Geometry: final body of the model. Coordinates: model frame, mm. A direction names the side the tool comes from. Give positions to 0.01 mm unless a question says otherwise; leave off trailing zeros. Order: outer loops, then holes, each group sorted by start corner. A loop starts at its lowest first (then second) coordinate and runs counter-clockwise, first axis right, second up. Notation, with made-up numbers: (58, 44.25) -> (65, 44.25) arc R14 cw to (65, 53.25) -> close; hole circle Ø4 at (76, 13.25). An arc over 180 degrees is marked (long way). One line per question, with ' | ' between items.
from build123d import *

# Parameters (mm, degrees)
BOSS_EXTRUDE1_DEPTH   = 3.175
BOSS_EXTRUDE1_2_DEPTH = 3.175
BOSS_EXTRUDE1_3_DEPTH = 3.175
BOSS_EXTRUDE1_4_DEPTH = 3.175
SKETCH1_R             = 3.2
SKETCH1_W             = 12.5
SKETCH1_H             = 20
BOSS_EXTRUDE1_5_DEPTH = 3.175
SKETCH2_W             = 43.267164734
SKETCH2_H             = 48
SKETCH2_W_2           = 36.488078293
BOSS_EXTRUDE2_DEPTH   = 3.175
SKETCH3_W             = 150
SKETCH3_H             = 50.164895034
SKETCH3_W_2           = 146
SKETCH3_H_2           = 48
BOSS_EXTRUDE3_DEPTH   = 3.175
SKETCH4_R             = 3.175
CUT_EXTRUDE1_DEPTH    = 3.175


with BuildPart() as part:
    # Sketch1 → Boss-Extrude1 (new body)
    with BuildSketch(Plane.XY):
        Polygon((57.693747285, -13.75), (57.693747285, -24), (73, -24), (73, -10.75), (53.098076211, -10.75), (53.098076211, -13.75), align=None)
    extrude(amount=BOSS_EXTRUDE1_DEPTH)



with BuildPart() as body_2:
    # Sketch1 → Boss-Extrude1 2 (new body)
    with BuildSketch(Plane.XY):
        Polygon((53.098076211, 13.25), (73, 13.25), (73, 24), (57.693747285, 24), (57.693747285, 16.25), (53.098076211, 16.25), align=None)
    extrude(amount=BOSS_EXTRUDE1_2_DEPTH)


with BuildPart() as body_3:
    # Sketch1 → Boss-Extrude1 3 (new body)
    with BuildSketch(Plane.XY):
        Polygon((-73, -10.75), (-73, -24), (-57.693747285, -24), (-57.693747285, -13.75), (-53.098076211, -13.75), (-53.098076211, -10.75), align=None)
    extrude(amount=BOSS_EXTRUDE1_3_DEPTH)


with BuildPart() as body_4:
    # Sketch1 → Boss-Extrude1 4 (new body)
    with BuildSketch(Plane.XY):
        Polygon((-57.693747285, 24), (-73, 24), (-73, 13.25), (-53.098076211, 13.25), (-53.098076211, 16.25), (-57.693747285, 16.25), align=None)
    extrude(amount=BOSS_EXTRUDE1_4_DEPTH)


with BuildPart() as body_5:
    # Sketch1 → Boss-Extrude1 5 (new body)
    with BuildSketch(Plane.XY):
        Polygon((-43.306252715, -13.75), (-43.306252715, -24), (43.306252715, -24), (43.306252715, -13.75), (47.901923789, -13.75), (47.901923789, -6.75), (47.33772234, -6.75), (47.33772234, 9.25), (47.901923789, 9.25), (47.901923789, 16.25), (43.306252715, 16.25), (43.306252715, 24), (-43.306252715, 24), (-43.306252715, 16.25), (-47.901923789, 16.25), (-47.901923789, 9.25), (-47.33772234, 9.25), (-47.33772234, -6.75), (-47.901923789, -6.75), (-47.901923789, -13.75), align=None)
        with Locations((4.144011572, 1)):
            Circle(SKETCH1_R, mode=Mode.SUBTRACT)
        with Locations((-13.75, 1)):
            Rectangle(SKETCH1_W, SKETCH1_H, mode=Mode.SUBTRACT)
    extrude(amount=BOSS_EXTRUDE1_5_DEPTH)


with BuildPart() as part_1:
    add(part.part)

    add(body_2.part)  # Boss-Extrude2 merges body 2

    add(body_3.part)  # Boss-Extrude2 merges body 3

    add(body_4.part)  # Boss-Extrude2 merges body 4

    add(body_5.part)  # Boss-Extrude2 merges body 5
    # Sketch2 → Boss-Extrude2 (add)
    with BuildSketch(Plane.XY.offset(3.175)):
        with Locations((-51.366417633, 0)):
            Rectangle(SKETCH2_W, SKETCH2_H)
        with Locations((54.755960853, 0)):
            Rectangle(SKETCH2_W_2, SKETCH2_H)
    extrude(amount=-BOSS_EXTRUDE2_DEPTH)

    # Sketch3 → Boss-Extrude3 (add)
    with BuildSketch(Plane.XY.offset(3.175)):
        with Locations((0, -0.917552483)):
            Rectangle(SKETCH3_W, SKETCH3_H)
        Rectangle(SKETCH3_W_2, SKETCH3_H_2, mode=Mode.SUBTRACT)
    extrude(amount=-BOSS_EXTRUDE3_DEPTH)

    # Sketch4 → Cut-Extrude1 (cut)
    with BuildSketch(Plane.XY.offset(3.175)):
        with Locations((-56.95575683, 12.857770953)):
            Circle(SKETCH4_R)
        with Locations((-44.95575683, 12.857770953)):
            Circle(SKETCH4_R)
        with Locations((-32.95575683, 12.857770953)):
            Circle(SKETCH4_R)
        with Locations((15.04424317, 12.857770953)):
            Circle(SKETCH4_R)
        with Locations((27.04424317, 12.857770953)):
            Circle(SKETCH4_R)
        with Locations((39.04424317, 12.857770953)):
            Circle(SKETCH4_R)
        with Locations((51.04424317, 12.857770953)):
            Circle(SKETCH4_R)
        with Locations((63.04424317, 12.857770953)):
            Circle(SKETCH4_R)
        with Locations((-62.280718202, 4.034960141)):
            Circle(SKETCH4_R)
        with Locations((-50.280718202, 4.034960141)):
            Circle(SKETCH4_R)
        with Locations((-38.280718202, 4.034960141)):
            Circle(SKETCH4_R)
        with Locations((21.719281798, 4.034960141)):
            Circle(SKETCH4_R)
        with Locations((33.719281798, 4.034960141)):
            Circle(SKETCH4_R)
        with Locations((45.719281798, 4.034960141)):
            Circle(SKETCH4_R)
        with Locations((57.719281798, 4.034960141)):
            Circle(SKETCH4_R)
        with Locations((-57.312596917, -4.551617996)):
            Circle(SKETCH4_R)
        with Locations((-45.312596917, -4.551617996)):
            Circle(SKETCH4_R)
        with Locations((-33.312596917, -4.551617996)):
            Circle(SKETCH4_R)
        with Locations((14.687403083, -4.551617996)):
            Circle(SKETCH4_R)
        with Locations((26.687403083, -4.551617996)):
            Circle(SKETCH4_R)
        with Locations((38.687403083, -4.551617996)):
            Circle(SKETCH4_R)
        with Locations((50.687403083, -4.551617996)):
            Circle(SKETCH4_R)
        with Locations((62.687403083, -4.551617996)):
            Circle(SKETCH4_R)
        with Locations((-62.637558288, -13.374428808)):
            Circle(SKETCH4_R)
        with Locations((-50.637558288, -13.374428808)):
            Circle(SKETCH4_R)
        with Locations((-38.637558288, -13.374428808)):
            Circle(SKETCH4_R)
        with Locations((-2.637558288, -13.374428808)):
            Circle(SKETCH4_R)
        with Locations((9.362441712, -13.374428808)):
            Circle(SKETCH4_R)
        with Locations((21.362441712, -13.374428808)):
            Circle(SKETCH4_R)
        with Locations((33.362441712, -13.374428808)):
            Circle(SKETCH4_R)
        with Locations((45.362441712, -13.374428808)):
            Circle(SKETCH4_R)
        with Locations((57.362441712, -13.374428808)):
            Circle(SKETCH4_R)
    extrude(amount=-CUT_EXTRUDE1_DEPTH, mode=Mode.SUBTRACT)


solid = part_1.part
1) Material intervals for probe 1 along Y at (x, z) = (-55.5, 1.5); probe 2 along X at (y, z) = (-0.5, 0.25); probe 3 along Y at (x, z) = (-61, 2.05), sorted ascending. Write a range as from..to.
Check result:
probe 1: y = -26..-7.16, -1.94..10.04, 15.68..24.16 | probe 2: x = -75..-20, -7.5..1.32, 6.97..75 | probe 3: y = -26..-16.09, -10.65..1.13, 6.94..24.16
2) Section B-B on x = 33.5. Return loops of the section in (y, z) (3 decimals).
Check result:
outline: (-26, 0) -> (-16.546, 0) -> (-16.546, 3.175) -> (-26, 3.175) -> close; (-10.202, 0) -> (0.868, 0) -> (0.868, 3.175) -> (-10.202, 3.175) -> close; (7.202, 0) -> (24.165, 0) -> (24.165, 3.175) -> (7.202, 3.175) -> close
3) Section C-C on z = 2.65. Count the separate pieces of the cut face and the enclosed holes in it, plus the area to 3 significant figures.
Check result:
separate pieces: 1 | enclosed holes: 34 | area: 6,230 mm^2
4) Set-up query: faces 4 (the flat face through (-1, -1, 0)), 5 (the flat face through (-14, -9, 2)). Return all of +Z, -Z, +X, -X, +Y, -Y with unobstructed straight access to the full face (end or side cutting, diameter ignored); none if empty.
Check result:
face 4: -Z, +X, -X, +Y, -Y | face 5: +Z, -Z
5) Section A-A on x = -45. Return loops of the section in (y, z) (3 decimals), plus the area to 3 significant figures.
Check result:
outline: (-26, 0) -> (-7.711, 0) -> (-7.711, 3.175) -> (-26, 3.175) -> close; (-1.392, 0) -> (9.683, 0) -> (9.683, 3.175) -> (-1.392, 3.175) -> close; (16.032, 0) -> (24.165, 0) -> (24.165, 3.175) -> (16.032, 3.175) -> close | area: 119 mm^2
6) Pull-direction query (X, two-part tool) for faces 1 (the cylindrical face through (59.872, 12.997, 1.61)), 2 (the flat face through (75, -1, 2)), 3 (the flat face through (-75, -1, 2)); classes: +X half, -X half, draft (parallel to the pull), parting line (faces both ways), or undercut.
Check result:
face 1: undercut | face 2: +X half | face 3: -X half
